The drawing under review shows one solid part. Ordinate dimensions are in mm from its lowest x, y, z. Coordinates: 2 decimals unless noted, no trailing zeros. Write each loop counter-clockwise with the first axis right and the second up, starting at its lowest first coordinate (ties: lowest second). Pieces come first, ordered by that corner, then holes. Notation, with made-up numbers: (-10, 30.5) - (18, 30.5) arc R29 ccw to (18, 63.5) - close; hole circle Ø11 at (59, 65). An arc over 180 degrees is marked (long way). Use a Markdown table: item, result.
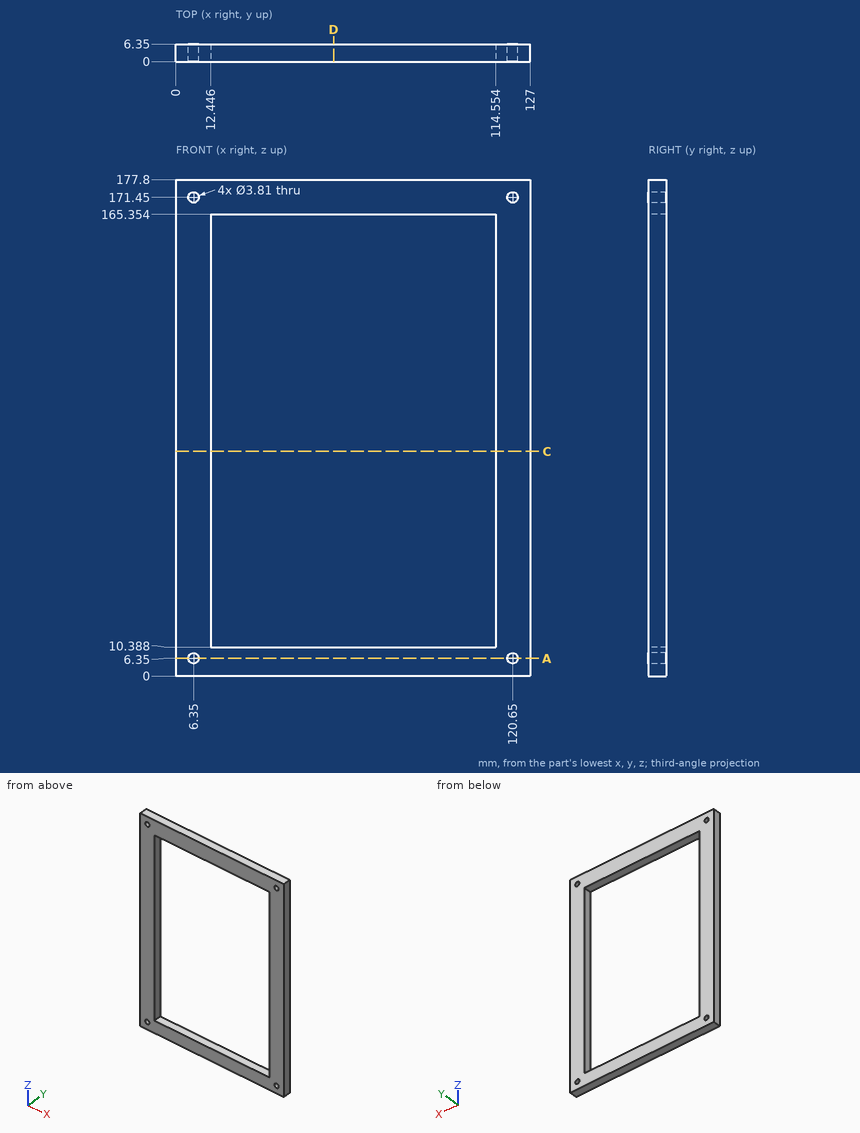
(1) Take a section at C-C on z = 80.5. Write out the cut boundary in (x, y), and give its area (3 significant figures).
Determined:
| item | result |
|---|---|
| outline | (0, 0) - (12.45, 0) - (12.45, 6.35) - (0, 6.35) - close; (114.55, 0) - (127, 0) - (127, 6.35) - (114.55, 6.35) - close |
| area | 158 mm2 |
(2) For pin 1 (12 mm diameter, centred on x = 68, z = 22, fed in from +Y); pin 2 (1 mm diameter, centred on x = 17.5, y = 4.5, fed in from -Z), all flat-tipped, find the tip position at first contact; note any pin that passes through.
Determined:
| item | result |
|---|---|
| pin 1 | through |
| pin 2 | z = 0 |
(3) Take a section at D-D on x = 56.5. Write out the cut boundary in (y, z).
Determined:
| item | result |
|---|---|
| outline | (0, 0) - (6.35, 0) - (6.35, 10.39) - (0, 10.39) - close; (0, 165.35) - (6.35, 165.35) - (6.35, 177.8) - (0, 177.8) - close |
(4) Take a section at A-A on z = 6.35. State how many separate pieces and enclosed holes the cut face has, and give its area (3 significant figures).
Determined:
| item | result |
|---|---|
| separate pieces | 3 |
| enclosed holes | 0 |
| area | 758 mm2 |
(5) For L1, parallel to X at y = 4.5, z = 6.35 (1 decimal); L2, parallel to X at y = 5.5, z = 56.5; L3, parallel to Z at x = 54, y = 3.75, list the stretches that pass through material, from the lowest coordinate up. Write a range as from..to.
Determined:
| item | result |
|---|---|
| L1 | 0..4.4, 8.3..118.7, 122.6..127 |
| L2 | 0..12.45, 114.55..127 |
| L3 | 0..10.39, 165.35..177.8 |
